Geometry: final body of the model. Coordinates: model frame, mm. A direction names the side the tool comes from. Give positions to 0.01 mm unless a question says otherwise; leave off trailing zeros. Write each loop counter-clockwise with the first axis right and the second up, starting at its lowest first coordinate (ties: lowest second). Pieces come first, ordered by that corner, then holes. Notation, with made-up numbers: (5.25, 53) -> (11.25, 53) arc R19 ccw to (11.25, 80) -> close; hole circle Ø10 at (15, 7.5). An arc over 180 degrees is marked (long way). Answer in a Markdown table with one row per item. Add a question column.
from build123d import *

# Parameters (mm, degrees)
F2_R     = 4.191
F3_DEPTH = 25.4


with BuildPart() as f1:
    # F0 (on Front) → F1 (revolve)
    with BuildSketch(Plane.XZ):
        Polygon((8.89, 6.35), (8.89, 0), (12.7, 0), (12.7, 8.255), (7.366, 13.7414), (7.366, 16.9164), (0, 16.9164), (0, 6.35), align=None)
    revolve(axis=Axis((0, 0, 11.6332), (0, 0, 1)))

    # F2 (on face) → F3 (cut)
    with BuildSketch(Plane.XY.offset(16.9164)):
        Circle(F2_R)
    extrude(amount=-F3_DEPTH, mode=Mode.SUBTRACT)


solid = f1.part
Q1. Pull-direction query (X, two-part tool) for faces 4 (the flat face through (3.2, -3.2, 16.916)), 5 (the conical face through (7.27, 2.29, 13.48)), 6 (the flat face through (-2, -4, 6.35)); classes: +X half, -X half, draft (parallel to the pull), parting line (faces both ways), or undercut.
Q2. Line query: probe 1 along Y at (x, z) = (0, 3.5); probe 2 along Y at (x, z) = (-0.5, 10); probe 3 along X at (y, z) = (-1.25, 4). Output: solid intervals per line, ascending. Write a range as from..to.
Q3. Section B-B on z = 5.5. Return loops of the section in (x, y).
Q4. Section A-A on x = 0. Return loops of the section in (y, z) (3 decimals), and give its area (3 significant figures).
Q5. Contact query for flat-ended pins moving along their axis: pin 1 Ø4 at (y, z) = (-4, 12) entering from -X; pin 2 Ø2 at (x, z) = (3.5, 7.5) entering from +Y; pin 3 Ø1 at (y, z) = (-5, 2.5) entering from +X. Output: stop coordinate, or through.
Q6. Section C-C on z = 11. Return loops of the section in (x, y), and give its area (3 significant figures).
Q7. Access query for faces 1 (the cylindrical face through (-1.93, -8.68, 3.13)), 2 (the flat face through (9, -3, 0)), 3 (the cylindrical face through (3.399, -6.535, 15.351)). Directions: +Z, -Z, +X, -X, +Y, -Y. A direction counts if a zero-diameter tool reaches every point of the face in a straight line with its end or side. Return the directions, or none.
Checks:
| question | item | result |
|---|---|---|
| 1 | face 4 | draft |
| 1 | face 5 | parting line |
| 1 | face 6 | undercut |
| 2 | probe 1 | -12.7..-8.89, 8.89..12.7 |
| 2 | probe 2 | -10.99..-4.16, 4.16..10.99 |
| 2 | probe 3 | -12.64..-8.8, 8.8..12.64 |
| 3 | outline | circle Ø25.4 at (0, 0); hole circle Ø17.78 at (0, 0) |
| 4 | outline | (-12.7, 0) -> (-8.89, 0) -> (-8.89, 6.35) -> (-4.191, 6.35) -> (-4.191, 16.916) -> (-7.366, 16.916) -> (-7.366, 13.741) -> (-12.7, 8.255) -> close; (4.191, 6.35) -> (8.89, 6.35) -> (8.89, 0) -> (12.7, 0) -> (12.7, 8.255) -> (7.366, 13.741) -> (7.366, 16.916) -> (4.191, 16.916) -> close |
| 4 | area | 165 mm^2 |
| 5 | pin 1 | x = -10.37 |
| 5 | pin 2 | y = 12.45 |
| 5 | pin 3 | x = 11.88 |
| 6 | outline | circle Ø20.06 at (0, 0); hole circle Ø8.38 at (0, 0) |
| 6 | area | 261 mm^2 |
| 7 | face 1 | -Z |
| 7 | face 2 | -Z, +X, -X, +Y, -Y |
| 7 | face 3 | +Z |
